Source: CAD feature listing. Evaluate the final solid. Frame: model axes, mm. A direction names the side the tool comes from. Round coordinates to 2 decimals unless told otherwise and drop trailing zeros. Write each loop counter-clockwise with the first axis right and the second up, starting at its lowest first coordinate (ties: lowest second). Pieces come first, ordered by that corner, then holes.
from build123d import *

# Parameters (mm, degrees)
FURO_ROSCADO_DE_M41_D           = 3.3
FURO_ROSCADO_DE_M41_DEPTH       = 11.5
FURO_ROSCADO_DE_M41_CSINK_D     = 4.05
FURO_ROSCADO_DE_M41_CSINK_ANGLE = 90
FURO_ROSCADO_DE_M41_TIP         = 0.991420021


with BuildPart() as part:
    # Esboço1 → Revolução1 (revolve)
    with BuildSketch(Plane.XY, mode=Mode.PRIVATE) as revolu_o1_sk:
        with BuildLine():
            Line((0, 0), (0, -16.5))
            Line((0, -16.5), (3.9, -16.5))
            Line((3.9, -16.5), (3.9, -2))
            Line((3.9, -2), (5, -2))
            ThreePointArc((5, -2), (9.419417382, -3.830582618), (11.25, -8.25))
            Line((11.25, -8.25), (13.25, -8.25))
            ThreePointArc((13.25, -8.25), (10.833630945, -2.416369055), (5, 0))
            Line((5, 0), (0, 0))
        make_face()
    revolve(revolu_o1_sk.sketch.rotate(Axis((0, 0, 0), (0, -1, 0)), 90), axis=Axis((0, 0, 0), (0, -1, 0)))

    # Furo roscado de M41
    with Locations(Plane(origin=(0, -16.5, 0), x_dir=(-1, 0, 0), z_dir=(0, -1, 0))):
        with Locations((0, 0)):
            CounterSinkHole(FURO_ROSCADO_DE_M41_D / 2, FURO_ROSCADO_DE_M41_CSINK_D / 2, depth=FURO_ROSCADO_DE_M41_DEPTH, counter_sink_angle=FURO_ROSCADO_DE_M41_CSINK_ANGLE)
            with Locations((0, 0, -(FURO_ROSCADO_DE_M41_DEPTH + FURO_ROSCADO_DE_M41_TIP / 2))):  # 118° drill point
                Cone(0, FURO_ROSCADO_DE_M41_D / 2, FURO_ROSCADO_DE_M41_TIP, mode=Mode.SUBTRACT)


solid = part.part
1) Pull-direction query (Z, two-part tool) for faces 1 (the face through (-0.1, -4.2, 0.3)), 2 (the face through (10, -8.25, 6)); classes: released by +Z, released by -Z, zero draft, split by the parting line, or undercut.
Taken from the geometry:
face 1: undercut
face 2: zero draft
2) Contact query for flat-ended pins moving along their axis: P1, Ø3, axis at x = 0, z = 0, coming from the -Y side; P2, Ø1.5, axis at x = 10, y = -7.5, coming from the +Z side; P3, Ø8, axis at y = -8, z = 8, coming from the +X side. Output: stop coordinate, or through.
Taken from the geometry:
P1: stops at y = -4.91
P2: stops at z = 9.44
P3: stops at x = 12.63
3) Material intervals for line 1 (X direction, y = -7, z = -1); line 2 (Z direction, x = 0.25, y = -6); line 3 (X direction, y = -11, z = 0.25), sorted ascending.
Taken from the geometry:
line 1: x = -13.12 to -11.08, -3.77 to -1.31, 1.31 to 3.77, 11.08 to 13.12
line 2: z = -12.93 to -10.83, -3.89 to -1.63, 1.63 to 3.89, 10.83 to 12.93
line 3: x = -3.89 to -1.63, 1.63 to 3.89
4) Reachability of faces 3 (the face through (2, -16.5, -2)), 4 (the face through (-2.64, -9.15, -2.87)) from +Z, -Z, +X, -X, +Y, -Y: full face, straight path, thin tool, end or side. Return the list, or none.
Taken from the geometry:
face 3: +Z, -Z, +X, -X, -Y
face 4: -Y
5) Section query B-B on y = -2.5. State how many separate pieces and enclosed holes the cut face has, then the cut area to 3 significant figures.
Taken from the geometry:
separate pieces: 2
enclosed holes: 1
area: 248 mm2
6) Section query A-A on y = -9.75. Return the cut outline in (x, z), then the cut area to 3 significant figures.
Taken from the geometry:
outline: circle Ø7.8 at (0, 0); hole circle Ø3.3 at (0, 0)
area: 39.2 mm2
